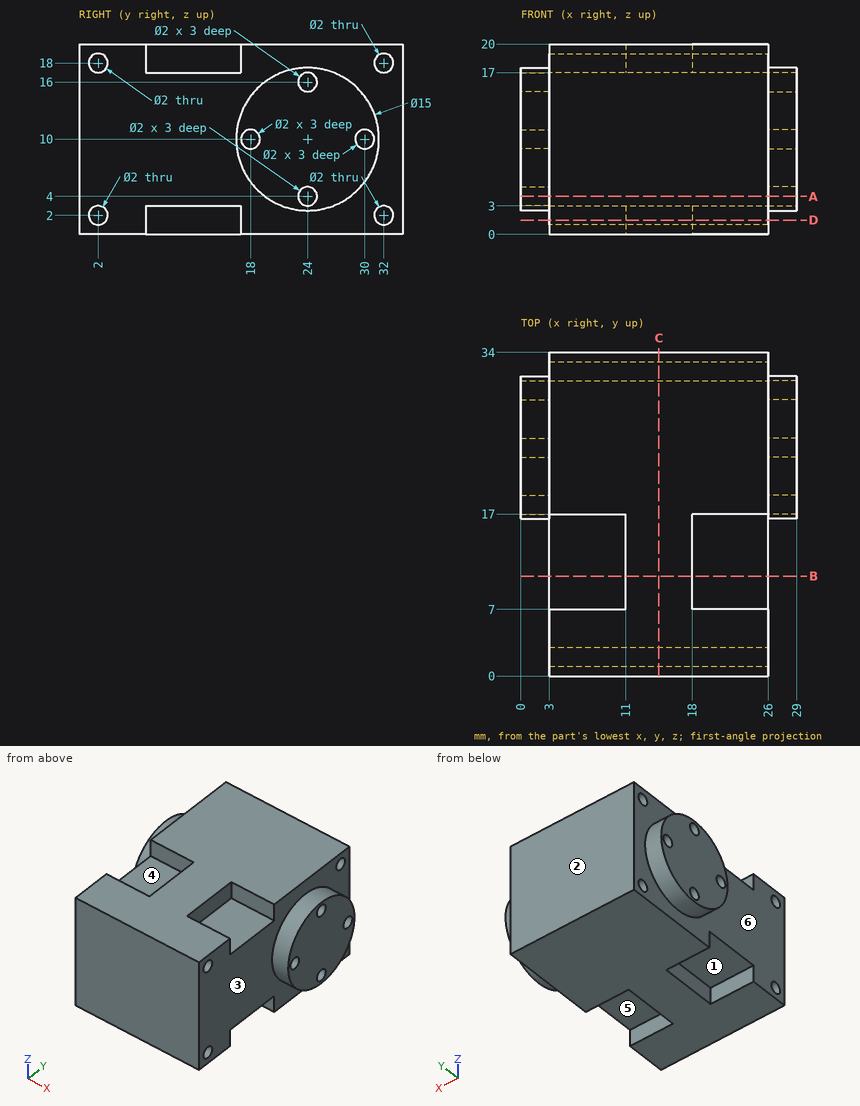
Study the drawing (mm; zero at the part's minimum x, y, z) and answer. A direction names the side the tool comes from. Give positions to 0.01 mm unless a question says otherwise; leave off trailing zeros. Loops run counter-clockwise (first coordinate to the right, second up) from the corner with the lowest first, then second, coordinate; pieces in that order, holes last. Notation, with made-up numbers: (61, -18.5) -> (118, -18.5) arc R14 ccw to (118, -10.5) -> close; hole circle Ø3 at (56, 70). An arc over 180 degrees is marked (long way). Use a Markdown table: item, result. Add a question column.
1) Which of the six approach directions +Z, -Z, +X, -X, +Y, -Y give full straight-line access (tool end or side, diameter ignored) to the marked faces 4, 5 and 6?
2) The part is cut by section C-C, the plane x = 14.5. Determine the outline of the cut face in (y, z), plus the area to 3 significant figures.
3) Consider line 1 along Z through (x, y) = (18.25, 32); line 2 along Y through (x, z) = (16.75, 18); line 3 along Y through (x, z) = (4, 1.5). Determine where each line is inside the solid, lowest interval first.
4) The part is cut by section D-D, the plane z = 1.5. Determine the outline of the cut face in (x, y).
5) For a pull along Y with two mould halves and no side action, classify the marked faces 1, 2 and 3 as +Y half, -Y half, draft (parallel to the pull), parting line (faces both ways), or undercut.
6) Each of these flat-tipped pins is pushed along its axis until it touches: P1, Ø0.9, axis at y = 10, z = 1.5, coming from the +X side; P2, Ø1.8, axis at y = 18, z = 10, coming from the -X side; P3, Ø0.9, axis at y = 13, z = 19, coming from the -X side. Where does it stop, or does it pass through?
7) The part is cut by section B-B, the plane y = 10.5. Determine the outline of the cut face in (x, z), plus the area to 3 significant figures.
8) The part is cut by section A-A, the plane z = 4. Determine the outline of the cut face in (x, y), plus the area to 3 significant figures.
Reported:
| question | item | result |
|---|---|---|
| 1 | face 4 | +Z, -X |
| 1 | face 5 | -Z, +X |
| 1 | face 6 | -X |
| 2 | outline | (0, 0) -> (34, 0) -> (34, 20) -> (0, 20) -> close; hole circle Ø2 at (2, 2); hole circle Ø2 at (2, 18); hole circle Ø2 at (32, 2); hole circle Ø2 at (32, 18) |
| 2 | area | 667 mm^2 |
| 3 | line 1 | z = 0 to 1, 3 to 17, 19 to 20 |
| 3 | line 2 | y = 0 to 1, 3 to 31, 33 to 34 |
| 3 | line 3 | y = 0 to 1.13, 2.87 to 7, 17 to 31.13, 32.87 to 34 |
| 4 | outline | (3, 0) -> (26, 0) -> (26, 1.13) -> (3, 1.13) -> close; (3, 2.87) -> (26, 2.87) -> (26, 7) -> (18, 7) -> (18, 17) -> (26, 17) -> (26, 31.13) -> (3, 31.13) -> (3, 17) -> (11, 17) -> (11, 7) -> (3, 7) -> close; (3, 32.87) -> (26, 32.87) -> (26, 34) -> (3, 34) -> close |
| 5 | face 1 | undercut |
| 5 | face 2 | +Y half |
| 5 | face 3 | draft |
| 6 | P1 | stops at x = 18 |
| 6 | P2 | stops at x = 3 |
| 6 | P3 | stops at x = 11 |
| 7 | outline | (3, 3) -> (11, 3) -> (11, 0) -> (18, 0) -> (18, 3) -> (26, 3) -> (26, 17) -> (18, 17) -> (18, 20) -> (11, 20) -> (11, 17) -> (3, 17) -> close |
| 7 | area | 364 mm^2 |
| 8 | outline | (0, 19.5) -> (3, 19.5) -> (3, 0) -> (26, 0) -> (26, 19.5) -> (29, 19.5) -> (29, 23) -> (26, 23) -> (26, 25) -> (29, 25) -> (29, 28.5) -> (26, 28.5) -> (26, 34) -> (3, 34) -> (3, 28.5) -> (0, 28.5) -> (0, 25) -> (3, 25) -> (3, 23) -> (0, 23) -> close |
| 8 | area | 824 mm^2 |
